The model under review builds one solid part; all positions refer to its coordinate system, in mm. A direction names the side the tool comes from. Round coordinates to 2 decimals unless told otherwise and drop trailing zeros. Order: outer loops, then holes, each group sorted by start corner. A loop starts at its lowest first (then second) coordinate and runs counter-clockwise, first axis right, second up. Notation, with made-up numbers: M -25.75,86 L 11.25,86 A18 ccw 11.25,116 Z; hole C -4,-7.5 d10. An arc over 180 degrees is marked long. Use a Markdown table: item, result. Add a question column.
1. Consider section D-D on x = 27.5. State the section outline as (y, z) points.
2. The part is to be moulded in two halves that separate along Z. For faces 1 (the flat face through (38.5, 13, 17)), 2 (the flat face through (20, 5, 0)), 3 (the flat face through (35, 10, 55)), say which applies: +Z half, -Z half, draft (parallel to the pull), parting line (faces both ways), or undercut.
3. Consider section A-A on z = 1.25. State the section outline as (x, y) points.
4. Consider section B-B on z = 9. State the section outline as (x, y) points.
5. To check wall thickness, follow probe 1 along X at (y, z) = (13.75, 33); probe 2 along X at (y, z) = (7.25, 11); probe 3 along Y at (x, z) = (40.55, 9). State the ranges of each line that lie inside material, in increasing order.
6. For faces 4 (the flat face through (13.5, 4.5, 24.8)), 5 (the cylindrical face through (39.979, 7.028, 7.566)), 6 (the flat face through (41.5, 10, 20)), 7 (the flat face through (66, 10, 0)), 8 (the cylindrical face through (6.656, 2.813, 19.296)), list the 3-axis set-ups (+Z, -Z, +X, -X, +Y, -Y) from which the entire face can be reached by the end or side of a thin tool; tool diameter is ignored.
7. Consider section C-C on y = 16. State the section outline as (x, z) points.
8. Insertion check: P1, Ø12, axis at y = 17.5, z = 25, coming from the -X side; P2, Ø2.5, axis at y = 6.58, z = 24.5, coming from the -X side; P3, Ø2.5, axis at x = 65.5, y = 12, coming from the -Z side. Each pin has a flat end and moves straight along its axis. Give the tip position at first contact, or say it passes through.
from build123d import *

# Parameters (mm, degrees)
SKETCH1_W           = 70
SKETCH1_H           = 55
BOSS_EXTRUDE1_DEPTH = 20
SKETCH2_R           = 26
CUT_EXTRUDE1_DEPTH  = 20.5
SKETCH3_R           = 17.5
CUT_EXTRUDE2_DEPTH  = 13.5
SKETCH5_R           = 19.5
CUT_EXTRUDE3_DEPTH  = 28
SKETCH6_R           = 1.503081696
BOSS_EXTRUDE2_DEPTH = 3


with BuildPart() as part:
    # Sketch1 → Boss-Extrude1 (new body)
    with BuildSketch(Plane(origin=(0, 0, 0), x_dir=(1, 0, 0), z_dir=(0, 1, 0))):
        with Locations((35, -27.5)):
            Rectangle(SKETCH1_W, SKETCH1_H)
    extrude(amount=BOSS_EXTRUDE1_DEPTH)

    # Sketch2 → Cut-Extrude1 (cut)
    with BuildSketch(Plane(origin=(62, 0, 0), x_dir=(0, 0, -1), z_dir=(1, 0, 0))):
        with Locations((-16, 20)):
            Circle(SKETCH2_R)
    extrude(amount=-CUT_EXTRUDE1_DEPTH, mode=Mode.SUBTRACT)

    # Sketch3 → Cut-Extrude2 (cut)
    with BuildSketch(Plane.ZY):
        with Locations((16, 20)):
            Circle(SKETCH3_R)
    extrude(amount=-CUT_EXTRUDE2_DEPTH, mode=Mode.SUBTRACT)

    # Sketch5 → Cut-Extrude3 (cut)
    with BuildSketch(Plane.ZY.offset(-13.5)):
        with Locations((16.75, 20)):
            Circle(SKETCH5_R)
    extrude(amount=-CUT_EXTRUDE3_DEPTH, mode=Mode.SUBTRACT)

    # Sketch6 → Boss-Extrude2 (add)
    with BuildSketch(Plane(origin=(38.5, 0, 0), x_dir=(0, 0, -1), z_dir=(1, 0, 0))):
        with BuildLine():
            Line((2.75, 20), (0.253081696, 20))
            ThreePointArc((0.253081696, 20), (-1.25, 18.496918304), (-2.753081696, 20))
            Line((-2.753081696, 20), (-30.746918304, 20))
            ThreePointArc((-30.746918304, 20), (-32.25, 18.496918304), (-33.753081696, 20))
            Line((-33.753081696, 20), (-36.25, 20))
            ThreePointArc((-36.25, 20), (-16.75, 0.5), (2.75, 20))
        make_face()
        with Locations((-9, 6.576606241)):
            Circle(SKETCH6_R, mode=Mode.SUBTRACT)
        with Locations((-24.5, 6.576606241)):
            Circle(SKETCH6_R, mode=Mode.SUBTRACT)
    extrude(amount=BOSS_EXTRUDE2_DEPTH)


solid = part.part
Answer block:
| question | item | result |
|---|---|---|
| 1 | outline | M 0,0 L 10.02,0 A19.5 cw 20,36.25 L 20,55 L 0,55 Z |
| 2 | face 1 | undercut |
| 2 | face 2 | -Z half |
| 2 | face 3 | +Z half |
| 3 | outline | M 0,0 L 41.5,0 L 41.5,18.5 L 38.5,18.5 L 38.5,8.17 L 13.5,8.17 L 13.5,10.58 L 0,10.58 Z; M 62,0 L 70,0 L 70,20 L 62,20 Z |
| 4 | outline | M 0,0 L 41.5,0 L 41.5,5.07 L 38.5,5.07 L 38.5,2.11 L 13.5,2.11 L 13.5,3.96 L 0,3.96 Z; M 38.5,8.08 L 41.5,8.08 L 41.5,20 L 38.5,20 Z; M 62,0 L 70,0 L 70,20 L 62,20 Z |
| 5 | probe 1 | 0 to 13.5, 38.5 to 41.5, 62 to 70 |
| 5 | probe 2 | 38.5 to 41.5, 62 to 70 |
| 5 | probe 3 | 0 to 5.07, 8.08 to 20 |
| 6 | face 4 | +Y |
| 6 | face 5 | -X |
| 6 | face 6 | -Z, +Y |
| 6 | face 7 | -Z, +X, +Y, -Y |
| 6 | face 8 | -X, +Y |
| 7 | outline | M 0,33.04 L 13.5,33.04 L 13.5,35.84 L 38.5,35.84 L 38.5,-2.34 L 41.5,-2.34 L 41.5,41.69 L 62,41.69 L 62,0 L 70,0 L 70,55 L 0,55 Z |
| 8 | P1 | x = 38.5 |
| 8 | P2 | x = 62 |
| 8 | P3 | z = 0 |
